Source: CAD feature listing. Evaluate the final solid. Frame: model axes, mm. Face numbers are marked on the shaded views. A direction names the side the tool comes from. Give positions to 0.01 mm unless a question says otherwise; leave off trailing zeros. Write each loop counter-clockwise with the first axis right and the second up, starting at its lowest first coordinate (ties: lowest second). Pieces come first, ordered by that corner, then holes. Notation, with made-up numbers: (-9, -21.75) -> (16, -21.75) arc R33 cw to (16, 7.25) -> close; hole circle Ø7 at (-37.75, -17.5). An arc over 180 degrees is marked (long way). Write item = value, one per line.
from build123d import *

# Parameters (mm, degrees)
SKETCH1_W           = 25.4
SKETCH1_H           = 3.81
SKETCH1_W_2         = 5.08
SKETCH1_H_2         = 1.524
BOSS_EXTRUDE1_DEPTH = 2.54
SKETCH3_W           = 15.24
SKETCH3_H           = 7.62
BOSS_EXTRUDE2_DEPTH = 4.572
SKETCH4_R           = 1.524
CUT_EXTRUDE1_DEPTH  = 21.358064348


with BuildPart() as part:
    # Sketch1 → Boss-Extrude1 (new body)
    with BuildSketch(Plane(origin=(0, 0, 0), x_dir=(1, 0, 0), z_dir=(0, 1, 0))):
        Rectangle(SKETCH1_W, SKETCH1_H)
        with Locations((8.052340426, 0)):
            Rectangle(SKETCH1_W_2, SKETCH1_H_2, mode=Mode.SUBTRACT)
    extrude(amount=BOSS_EXTRUDE1_DEPTH)

    # Sketch3 → Boss-Extrude2 (add)
    with BuildSketch(Plane(origin=(12.7, 0, 0), x_dir=(0, 0, -1), z_dir=(1, 0, 0))):
        with Locations((0, 2.602908147)):
            Rectangle(SKETCH3_W, SKETCH3_H)
    extrude(amount=BOSS_EXTRUDE2_DEPTH)

    # Sketch4 → Cut-Extrude1 (cut, through all)
    with BuildSketch(Plane(origin=(0, 6.412908147, 0), x_dir=(1, 0, 0), z_dir=(0, 1, 0))):
        with Locations(Location((14.879777227, -5.08, 0), (0, 0, 270))):
            Circle(SKETCH4_R)
        with Locations(Location((14.879777227, 5.08, 0), (0, 0, 90))):
            Circle(SKETCH4_R)
    extrude(amount=-CUT_EXTRUDE1_DEPTH, mode=Mode.SUBTRACT)


solid = part.part
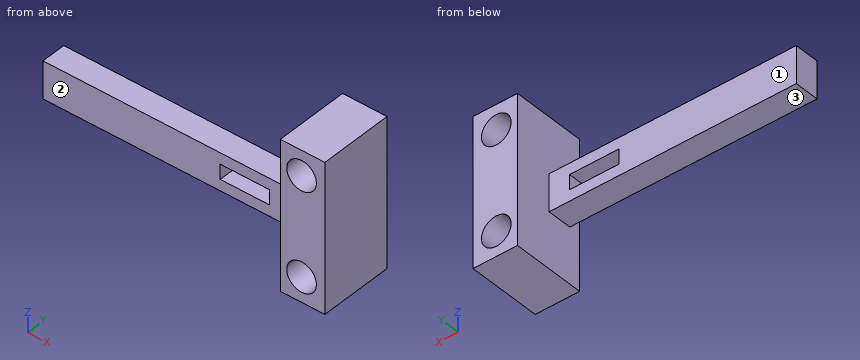
1) Cut plane B-B (x = 9.25). Return the cut outline in (y, z) (3 decimals), then the cut area to 3 significant figures.
Computed:
outline = (0, -1.905) -> (2.54, -1.905) -> (2.54, -0.762) -> (0, -0.762) -> close; (0, 0.762) -> (2.54, 0.762) -> (2.54, 1.905) -> (0, 1.905) -> close
area = 5.81 mm²
2) Contact query for flat-ended pins moving along their axis: pin 1 (3 mm diameter, centred on x = -1.5, z = 1, fed in from -Y); pin 2 (1.3 mm diameter, centred on x = 8, y = 0.5, fed in from -Z) (3 decimals); pin 3 (1.3 mm diameter, centred on x = 7, y = 1.5, fed in from +Z) (3 decimals); pin 4 (2 mm diameter, centred on x = 3, y = 4.5, fed in from -Z). Output: stop coordinate, or through.
Computed:
pin_1 = 0
pin_2 = -1.905
pin_3 = 1.905
pin_4 = through
3) Cut plane D-D (x = -5.5). Return the cut outline in (y, z) (3 decimals), then the cut area to 3 significant figures.
Computed:
outline = (0, -1.905) -> (2.54, -1.905) -> (2.54, 1.905) -> (0, 1.905) -> close
area = 9.68 mm²
4) Material intervals for L1, parallel to X at y = 2.25, z = 5.08; L2, parallel to Z at x = 9.5, y = 1 (3 decimals); L3, parallel to Z at x = 14, y = 4.5, sorted ascending.
Computed:
L1 = 12.7 to 13.36, 16.4 to 17.27
L2 = -1.905 to -0.762, 0.762 to 1.905
L3 = -7.62 to -6.32, -3.84 to 3.84, 6.32 to 7.62
5) Cut plane A-A (z = -5.08). Return the cut outline in (x, y).
Computed:
outline = (12.7, -1.21) -> (13.36, -1.21) -> (13.36, 6.41) -> (12.7, 6.41) -> close; (16.4, -1.21) -> (17.27, -1.21) -> (17.27, 6.41) -> (16.4, 6.41) -> close
6) Access query for the marked faces 1, 2 and 3. Directions: +Z, -Z, +X, -X, +Y, -Y. A direction counts if a zero-diameter tool reaches every point of the face in a straight line with its end or side. Return the directions, or none.
Computed:
face_1 = +Z, -Z, -X, +Y
face_2 = +Z, -Z, -X, -Y
face_3 = -Z, -X, +Y, -Y
7) Cut plane C-C (y = 4). Return the cut outline in (x, z).
Computed:
outline = (12.7, -7.62) -> (17.27, -7.62) -> (17.27, 7.62) -> (12.7, 7.62) -> close; hole circle Ø3.05 at (14.88, -5.08); hole circle Ø3.05 at (14.88, 5.08)
